Input: part model. Units: mm. Frame: model coordinates. Face numbers are marked on the shaded views. Round coordinates to 2 decimals unless told otherwise and drop trailing zeros. Order: outer loops, then holes, each group sorted by start corner. A loop starts at its lowest first (then second) coordinate and runs counter-clockwise, first axis right, second up. Notation, with made-up numbers: (-35, 32) - (0, 32) arc R3 cw to (0, 36) - close; hole circle Ø8 at (-20, -15.5). An arc over 180 degrees is marked (long way). One line per item, written item: value. Start each with the question number.
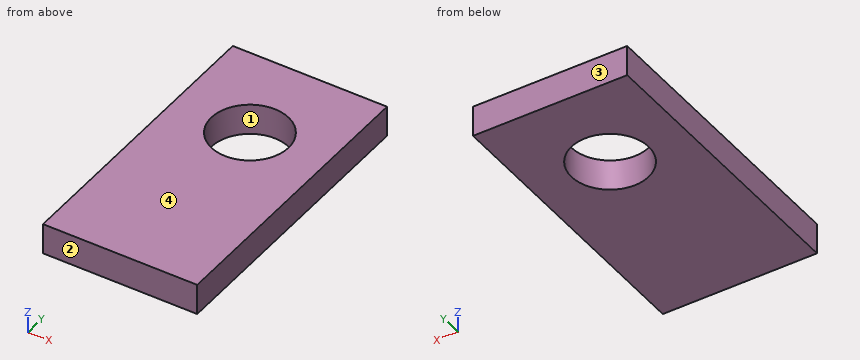
Autodesk Inventor part; units mm, degrees
ref_plane "YZ Plane" through (0, 0, 0) normal (1, 0, 0) x (0, 1, 0)
ref_plane "XZ Plane" through (0, 0, 0) normal (0, 1, 0) x (-1, 0, 0)
ref_plane "XY Plane" through (0, 0, 0) normal (0, 0, 1) x (1, 0, 0)
sketch "Boceto1" plane through (0, 0, 0) normal (0, 0, 1) x (1, 0, 0)
  line L0 (0, 0) -> (50, 0)
  line L1 (50, 0) -> (50, -95)
  line L2 (50, -95) -> (0, -95)
  line L3 (0, -95) -> (0, 0)
  circle A0 centre (25, -30) radius 12.5
  dimension "d0" = 50
  dimension "d1" = 95
  dimension "d2" = 25
extrude "Extrusión1" add sketch "Boceto1" along normal blind 10
properties part number "BaseM"
Item 1: First-contact query: pin 1 Ø8 at (x, y) = (29.5, -36.5) entering from -Z. Flat tip, straight axial feed; report the tip coordinate or a pass-through.
Item 2: Line query: L1, parallel to Y at x = 25, z = 4; L2, parallel to Y at x = 14, z = 0.5; L3, parallel to X at y = -19.5, z = 8.75. Output: solid intervals per line, ascending.
Item 3: Section query A-A on y = -30. Return loops of the section in (x, z).
Item 4: Section query C-C on z = 5.5. Return loops of the section in (x, y), and give its area (3 significant figures).
Item 5: Section query B-B on x = 25. Return loops of the section in (y, z), and give its area (3 significant figures).
Item 6: Pull-direction query (Y, two-part tool) for the marked faces 1, 2, 3 and 4; classes: released by +Y, released by -Y, zero draft, split by the parting line, or undercut.
Geometry results:
1. pin 1: passes through
2. L1: y = -95 to -42.5, -17.5 to 0
2. L2: y = -95 to -35.94, -24.06 to 0
2. L3: x = 0 to 18.22, 31.78 to 50
3. outline: (0, 0) - (12.5, 0) - (12.5, 10) - (0, 10) - close; (37.5, 0) - (50, 0) - (50, 10) - (37.5, 10) - close
4. outline: (0, -95) - (50, -95) - (50, 0) - (0, 0) - close; hole circle Ø25 at (25, -30)
4. area: 4,260 mm^2
5. outline: (-95, 0) - (-42.5, 0) - (-42.5, 10) - (-95, 10) - close; (-17.5, 0) - (0, 0) - (0, 10) - (-17.5, 10) - close
5. area: 700 mm^2
6. face 1: undercut
6. face 2: released by -Y
6. face 3: released by +Y
6. face 4: zero draft
